from build123d import *

# Parameters (mm, degrees)
SKETCH_1_W       = 20
SKETCH_1_H       = 16
SKETCH_1_W_2     = 28
SKETCH_1_H_2     = 29
EXTRUDE_1_DEPTH  = 580
CHAMFER_1_SIZE   = 10
M10X1_25_1_D     = 8.8
M10X1_25_1_DEPTH = 59
M10X1_25_1_TIP   = 2.643786724
FILLET_1_R       = 5


with BuildPart() as part:
    # 草圖1 → 填料-伸長1 (new body)
    with BuildSketch(Plane(origin=(0, 0, 0), x_dir=(0, 0, -1), z_dir=(1, 0, 0))):
        Polygon((0, 60), (0, 45), (20, 45), (28, 45), (28, 60), align=None)
        with Locations((10, 37)):
            Rectangle(SKETCH_1_W, SKETCH_1_H)
        with Locations((14, 14.5)):
            Rectangle(SKETCH_1_W_2, SKETCH_1_H_2)
    extrude(amount=EXTRUDE_1_DEPTH)

    # 導角1
    chamfer_1_edges = [part.edges().sort_by_distance(p)[0] for p in [
        (290, 0, -28),
    ]]
    chamfer(chamfer_1_edges, length=CHAMFER_1_SIZE)

    # M10x1.25 螺紋孔1
    with Locations(Plane(origin=(0, 0, -20), x_dir=(-1, 0, 0), z_dir=(0, 0, -1))):
        with Locations((-555, 37), (-422.5, 37), (-290, 37), (-157.5, 37), (-25, 37)):
            Hole(M10X1_25_1_D / 2, depth=M10X1_25_1_DEPTH)
            with Locations((0, 0, -(M10X1_25_1_DEPTH + M10X1_25_1_TIP / 2))):  # 118° drill point
                Cone(0, M10X1_25_1_D / 2, M10X1_25_1_TIP, mode=Mode.SUBTRACT)

    # 圓角1
    fillet_1_edges = [part.edges().sort_by_distance(p)[0] for p in [
        (290, 0, 0),
    ]]
    fillet(fillet_1_edges, radius=FILLET_1_R)


solid = part.part
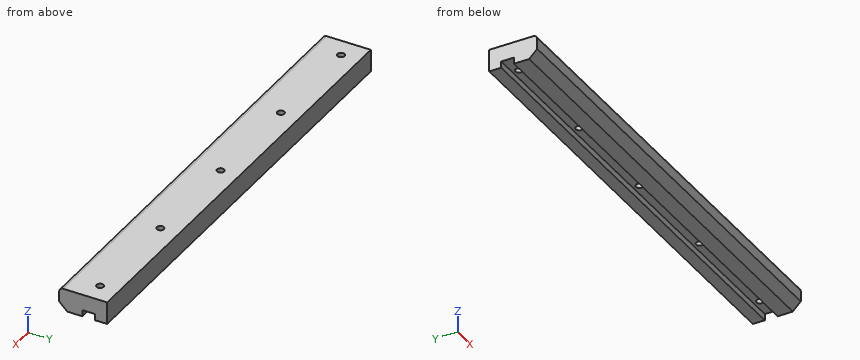
The listing builds one solid part. Answer for the finished solid, in the listing's coordinates (mm). Give positions to 0.01 mm unless a question says otherwise; leave off trailing zeros. Order: outer loops, then holes, each group sorted by start corner. A loop starts at its lowest first (then second) coordinate and runs counter-clockwise, first axis right, second up. Notation, with made-up numbers: (-30, 36) - (9, 36) arc R25 cw to (9, 64) - close; hole circle Ø10 at (79, -28). An arc over 180 degrees is marked (long way). Use one line per item in the form item = value.
1) Consider probe 1 along X at (y, z) = (33, -13.5); probe 2 along Y at (x, z) = (555, -15.5); probe 3 along X at (y, z) = (34, -16.5). Determine where each line is inside the solid, lowest interval first. Write a range as [from, to].
Verdict:
probe_1 = [0, 23.17], [26.83, 155.67], [159.33, 288.17], [291.83, 420.67], [424.33, 553.17], [556.83, 580]
probe_2 = [0, 32.6], [41.4, 60]
probe_3 = [0, 21.78], [28.22, 154.28], [160.72, 286.78], [293.22, 419.28], [425.72, 551.78], [558.22, 580]
2) Find section A-A on x = 63.5. Determine the outline of the cut face in (y, z), and give its area (3 significant figures).
Verdict:
outline = (0, -18) - (10, -28) - (29, -28) - (29, -20) - (45, -20) - (45, -28) - (60, -28) - (60, 0) - (5, 0) arc R5 ccw to (0, -5) - close
area = 1,500 mm^2
3) Each of these flat-tipped pins is pushed along its axis until it touches: pin 1 (6 mm diameter, centred on x = 181.5, z = -24, fed in from -Y); pin 2 (11.5 mm diameter, centred on x = 422.5, y = 37, fed in from -Z); pin 3 (6.5 mm diameter, centred on x = 254, z = -23.5, fed in from -Y). Where does it stop, or does it pass through?
Verdict:
pin_1 = 3
pin_2 = -20
pin_3 = 2.25
